Drawing for the job (mm, zero at the part's lowest x, y, z). Give positions to 0.01 mm unless a question says otherwise; leave off trailing zeros. Order: outer loops, then holes, each group sorted by start corner. A loop starts at its lowest first (then second) coordinate and runs counter-clockwise, first axis right, second up. Notation, with made-up numbers: (-30.5, -18.75) - (-13.5, -18.75) arc R23 cw to (-13.5, 11.25) - close; hole circle Ø10 at (-2.75, -20). An arc over 180 degrees is marked (long way). Use a Markdown table: item, result.
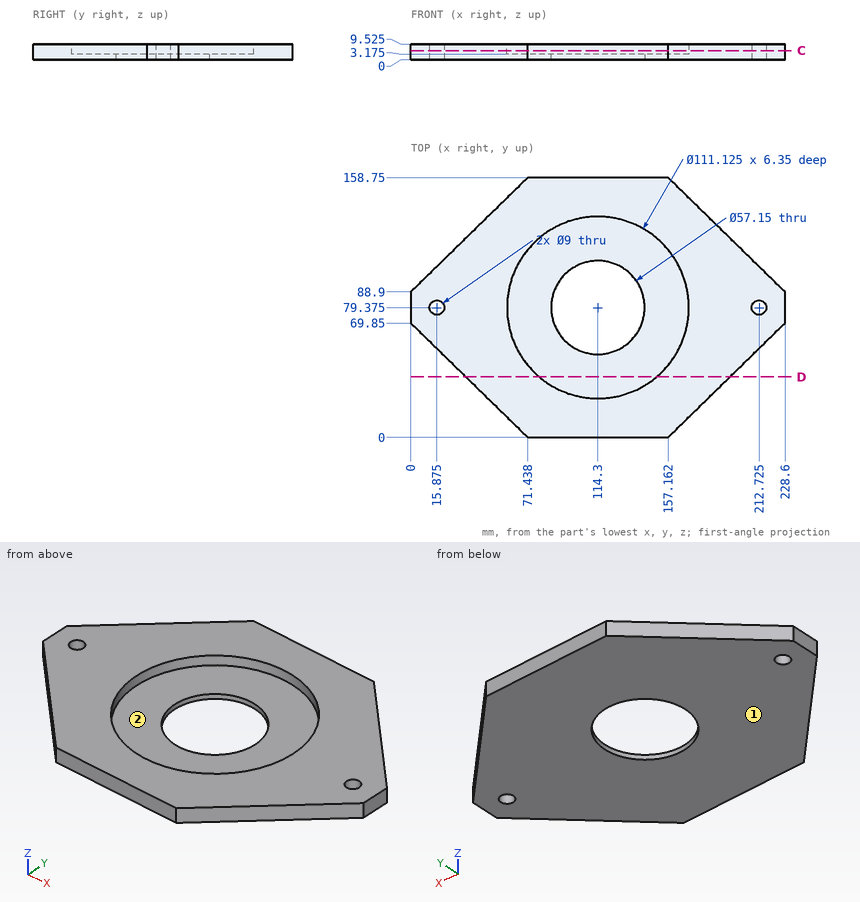
1) Pin check, flat tips, straight feed: P1, Ø5, axis at y = 56.5, z = 8.5, coming from the -X side (1 decimal); P2, Ø1.5, axis at x = 28.5, z = 5.5, coming from the +Y side; P3, Ø1.5, axis at x = 197, z = 5, coming from the +Y side; P4, Ø8, axis at x = 212.725, y = 79.375, coming from the -Z side. Stop position of each tip, or through.
Computed:
| item | result |
|---|---|
| P1 | stops at x = 11.1 |
| P2 | stops at y = 117.5 |
| P3 | stops at y = 120.53 |
| P4 | passes through |
2) Wall check: line 1 (Y direction, x = 114.3, z = 5.5); line 2 (Z direction, x = 144.5, y = 78) (1 decimal); line 3 (X direction, y = 60.5, z = 9.25) (1 decimal). Give the ranges that are in metal, low to high. Write a range as from..to.
Computed:
| item | result |
|---|---|
| line 1 | y = 0..23.81, 134.94..158.75 |
| line 2 | z = 0..3.2 |
| line 3 | x = 9.6..62, 166.6..219 |
3) Slice it at C-C (z = 5.5). State how many separate pieces and enclosed holes the cut face has, and give its area (3 significant figures).
Computed:
| item | result |
|---|---|
| separate pieces | 1 |
| enclosed holes | 3 |
| area | 16,500 mm² |
4) Two-plate mould, pull along X, no slides. Class the marked faces 1 and 2: +X half, -X half, draft (parallel to the pull), parting line (faces both ways), or undercut.
Computed:
| item | result |
|---|---|
| face 1 | draft |
| face 2 | undercut |
5) Slice it at D-D (y = 37). Write the cut outline in (x, z) (1 decimal).
Computed:
| item | result |
|---|---|
| outline | (33.6, 0) - (195, 0) - (195, 9.5) - (150.2, 9.5) - (150.2, 3.2) - (78.4, 3.2) - (78.4, 9.5) - (33.6, 9.5) - close |
